from build123d import *

# Parameters (mm, degrees)
F0_W     = 124
F0_H     = 46.5
F0_R     = 0.85
F0_R_2   = 2.5
F0_R_3   = 8.05
F1_DEPTH = 2.5


with BuildPart() as f1:
    # F0 (on Front) → F1 (new body)
    with BuildSketch(Plane.XZ):
        with Locations((65, 26.25)):
            Rectangle(F0_W, F0_H)
        with Locations((67.88, 25.46)):
            Circle(F0_R, mode=Mode.SUBTRACT)
        Polygon((84.29, 24.16), (84.29, 26.96), (89.29, 26.96), (94.29, 26.96), (94.29, 24.16), (89.29, 24.16), align=None, mode=Mode.SUBTRACT)
        with Locations((110.7, 25.46)):
            Circle(F0_R, mode=Mode.SUBTRACT)
        with Locations((18, 39.5)):
            Circle(F0_R_2, mode=Mode.SUBTRACT)
        with Locations((76.29, 34.33)):
            Circle(F0_R_3, mode=Mode.SUBTRACT)
        with Locations((102.29, 34.33)):
            Circle(F0_R_3, mode=Mode.SUBTRACT)
        with Locations((67.88, 43.2)):
            Circle(F0_R, mode=Mode.SUBTRACT)
        Polygon((83.49, 39.7), (83.49, 44.5), (89.29, 44.5), (95.09, 44.5), (95.09, 39.7), (89.29, 39.7), align=None, mode=Mode.SUBTRACT)
        with Locations((110.7, 43.2)):
            Circle(F0_R, mode=Mode.SUBTRACT)
    extrude(amount=F1_DEPTH)


solid = f1.part
The model under review builds one solid part; all positions refer to its coordinate system, in mm. A direction names the side the tool comes from. Give positions to 0.01 mm unless a question says otherwise; leave off trailing zeros. Order: outer loops, then holes, each group sorted by start corner. A loop starts at its lowest first (then second) coordinate and runs counter-clockwise, first axis right, second up. Notation, with made-up numbers: M -21,56 L 5,56 A30 ccw 5,95 Z; hole C 16.5,-5.75 d10. An arc over 180 degrees is marked long. Use one line per item in the form item = value. Start each with the question number.
Item 1: We need section C-C on x = 18. Give the boundary of the cut face in (y, z), plus the area to 3 significant figures.
Item 2: We need section B-B on y = -1.95. Give the number of separate pieces and of enclosed holes in the cut face, plus the area to 3 significant figures.
Item 3: To check wall thickness, follow line 1 along Z through (x, y) = (92.5, -1.55); line 2 along Z through (x, y) = (68, -2); line 3 along X through (y, z) = (-1.9, 43.2). State the ranges of each line that lie inside material, in increasing order. Write a range as from..to.
Item 4: We need section D-D on x = 76.29. Give the boundary of the cut face in (y, z).
Item 5: For faces 1 (the flat face through (84.29, -1, 26)), 2 (the flat face through (64, -2.5, 27)), list the 3-axis set-ups (+Z, -Z, +X, -X, +Y, -Y) from which the entire face can be reached by the end or side of a thin tool; tool diameter is ignored.
Item 6: The part is to be moulded in two halves that separate along X. For faces 3 (the flat face through (83.49, -1, 42)), 4 (the flat face through (89, -1, 39.7)), 5 (the flat face through (127, -1, 26)), 6 (the flat face through (64, 0, 27)), say which applies: pulls with the +X half, pulls with the -X half, needs draft (parallel to the pull), parting line crosses it, or undercut.
Item 7: We need section A-A on z = 34.33. Give the boundary of the cut face in (x, y), plus the area to 4 significant figures.
Completed:
q1.outline = M -2.5,3 L 0,3 L 0,37 L -2.5,37 Z; M -2.5,42 L 0,42 L 0,49.5 L -2.5,49.5 Z
q1.area = 104 mm²
q2.separate_pieces = 1
q2.enclosed_holes = 9
q2.area = 5,250 mm²
q3.line_1 = 3..24.16, 26.96..39.7, 44.5..49.5
q3.line_2 = 3..24.62, 26.3..42.36, 44.04..49.5
q3.line_3 = 3..67.03, 68.73..83.49, 95.09..109.85, 111.55..127
q4.outline = M -2.5,3 L 0,3 L 0,26.28 L -2.5,26.28 Z; M -2.5,42.38 L 0,42.38 L 0,49.5 L -2.5,49.5 Z
q5.face_1 = +Y, -Y
q5.face_2 = +Z, -Z, +X, -X, -Y
q6.face_3 = undercut
q6.face_4 = undercut
q6.face_5 = pulls with the +X half
q6.face_6 = needs draft
q7.outline = M 3,-2.5 L 68.24,-2.5 L 68.24,0 L 3,0 Z; M 84.34,-2.5 L 94.24,-2.5 L 94.24,0 L 84.34,0 Z; M 110.34,-2.5 L 127,-2.5 L 127,0 L 110.34,0 Z
q7.area = 229.5 mm²
